from build123d import *

# Parameters (mm, degrees)
SKETCH1_W           = 43.9
SKETCH1_H           = 22.45
SKETCH1_W_2         = 39.9
SKETCH1_H_2         = 18.45
SKETCH4_W           = 10.037411494
SKETCH4_H           = 9.392939089
BOSS_EXTRUDE2_DEPTH = 6
SKETCH4_3_R         = 2
CUT_EXTRUDE1_DEPTH  = 6


with BuildPart() as part:
    # Sweep1: sweep along a path in Sketch3
    with BuildLine(Plane(origin=(0, 0, 0), x_dir=(1, 0, 0), z_dir=(0, 1, 0))) as sweep1_path:
        Line((-2.386481251, 0), (-2.386481251, 18.515328192))
        ThreePointArc((-2.386481251, 18.515328192), (-1.420266616, 29.239701623), (1.447258265, 39.618673501))
        Line((1.447258265, 39.618673501), (16.488375541, 79.650398262))
        ThreePointArc((16.488375541, 79.650398262), (19.355900422, 90.02937014), (20.322115057, 100.753743571))
        Line((20.322115057, 100.753743571), (20.322115057, 130))
    # Sketch1 → Sweep1 (sweep)
    with BuildSketch(Plane.XY):
        with Locations((-2.386481251, 2.5875622)):
            Rectangle(SKETCH1_W, SKETCH1_H)
        with Locations((-2.386481251, 2.5875622)):
            Rectangle(SKETCH1_W_2, SKETCH1_H_2, mode=Mode.SUBTRACT)
    sweep(path=sweep1_path.line)

    # Sketch4 → Boss-Extrude2 (add)
    with BuildSketch(Plane(origin=(0, 13.8125622, 0), x_dir=(1, 0, 0), z_dir=(0, 1, 0))):
        with Locations((20.322115057, 125.303530456)):
            Rectangle(SKETCH4_W, SKETCH4_H)
    extrude(amount=-BOSS_EXTRUDE2_DEPTH)

    # Sketch4_3 → Cut-Extrude1 (cut)
    with BuildSketch(Plane(origin=(0, 13.8125622, 0), x_dir=(1, 0, 0), z_dir=(0, 1, 0))):
        with Locations(Location((20.322115057, 125.5, 0), (0, 0, 270))):
            Circle(SKETCH4_3_R)
    extrude(amount=-CUT_EXTRUDE1_DEPTH, mode=Mode.SUBTRACT)


solid = part.part
Design review of the part built by this model. Coordinates are the model's own, in mm. A direction names the side the tool comes from. Coordinates: 2 decimals unless noted, no trailing zeros. Order: outer loops, then holes, each group sorted by start corner. A loop starts at its lowest first (then second) coordinate and runs counter-clockwise, first axis right, second up.
Item 1: Take a section at B-B, the plane z = -109.5. Write out the cut boundary in (x, y).
Item 2: Take a section at A-A, the plane y = 6.5. Write out the cut boundary in (x, z), then the cut area to 3 significant figures.
Item 3: For pin 1 Ø4.5 at (y, z) = (10.5, -123.5) entering from -X; pin 2 Ø2 at (y, z) = (10.5, -83.5) entering from -X; pin 3 Ø12 at (x, y) = (31.5, 9.5) entering from -Z; pin 4 Ø5.5 at (y, z) = (-2, -9) entering from +X, all flat-tipped, find the tip position at first contact; note any pin that passes through.
Item 4: The part is to be moulded in two halves that separate along X. For faces 6 (the flat face through (-24.336, 3, -9)), 7 (the cylindrical face through (18.19, 2.46, -25.57)), 8 (the flat face through (29.62, 2.43, -52.19)), say which applies: pulls with the +X half, pulls with the -X half, needs draft (parallel to the pull), parting line crosses it, or undercut.
Item 5: For line 1 (X direction, y = 11.6, z = -125.5); line 2 (Y direction, x = 13, z = -88.5); line 3 (X direction, y = 2, z = -122), list the stretches that pass through material, from the lowest coordinate up.
Item 6: For faces 1 (the cylindrical face through (-21.085, 2.717, -32.608)), 2 (the flat face through (15.303, 10, -125)), 3 (the flat face through (20, 7.813, -123)), 4 (the flat face through (-1.628, 3, -116)), 5 (the flat face through (20, 10, -120.607)), list the 3-axis set-ups (+Z, -Z, +X, -X, +Y, -Y) from which the entire face can be reached by the end or side of a thin tool; tool diameter is ignored.
Item 7: Take a section at C-C, the plane x = 5.5. Write out the cut boundary in (y, z), then the cut area to 3 significant figures.
Item 8: Take a section at D-D, the plane z = -125.5. Write out the cut boundary in (x, y).
The answers:
1. outline: (-1.63, -8.64) - (42.27, -8.64) - (42.27, 13.81) - (-1.63, 13.81) - close; hole (0.37, -6.64) - (40.27, -6.64) - (40.27, 11.81) - (0.37, 11.81) - close
2. outline: (-24.34, -18.52) arc R81.95 ccw to (-19.1, -47.34) - (-4.06, -87.37) arc R38.05 cw to (-1.63, -100.75) - (-1.63, -130) - (0.37, -130) - (0.37, -100.75) arc R40.05 ccw to (-2.19, -86.67) - (-17.23, -46.64) arc R79.95 cw to (-22.34, -18.52) - (-22.34, 0) - (-24.34, 0) - close; (17.56, -18.52) arc R40.05 ccw to (20.12, -32.6) - (35.16, -72.63) arc R79.95 cw to (40.27, -100.75) - (40.27, -130) - (42.27, -130) - (42.27, -100.75) arc R81.95 ccw to (37.04, -71.93) - (21.99, -31.9) arc R38.05 cw to (19.56, -18.52) - (19.56, 0) - (17.56, 0) - close
2. area: 535 mm2
3. pin 1: stops at x = -1.63
3. pin 2: stops at x = -5.89
3. pin 3: stops at z = -130
3. pin 4: stops at x = 19.56
4. face 6: pulls with the -X half
4. face 7: undercut
4. face 8: pulls with the +X half
5. line 1: x = -1.63 to 0.37, 15.3 to 18.32, 22.32 to 25.34, 40.27 to 42.27
5. line 2: y = -8.64 to -6.64, 11.81 to 13.81
5. line 3: x = -1.63 to 0.37, 40.27 to 42.27
6. face 1: +Z
6. face 2: +Z, -Z
6. face 3: -Z
6. face 4: -Z, -X, +Y, -Y
6. face 5: none
7. outline: (-8.64, -130) - (-6.64, -130) - (-6.64, 0) - (-8.64, 0) - close; (11.81, -130) - (13.81, -130) - (13.81, 0) - (11.81, 0) - close
7. area: 520 mm2
8. outline: (-1.63, -8.64) - (42.27, -8.64) - (42.27, 13.81) - (22.32, 13.81) - (22.32, 7.81) - (25.34, 7.81) - (25.34, 11.81) - (40.27, 11.81) - (40.27, -6.64) - (0.37, -6.64) - (0.37, 11.81) - (15.3, 11.81) - (15.3, 7.81) - (18.32, 7.81) - (18.32, 13.81) - (-1.63, 13.81) - close
